Autodesk Inventor part; units mm, degrees
ref_plane "YZ Plane" through (0, 0, 0) normal (1, 0, 0) x (0, 1, 0)
ref_plane "XZ Plane" through (0, 0, 0) normal (0, 1, 0) x (-1, 0, 0)
ref_plane "XY Plane" through (0, 0, 0) normal (0, 0, 1) x (1, 0, 0)
sketch "Sketch1" plane through (0, 0, 0) normal (1, 0, 0) x (0, 1, 0)
  arc A0 (8.8122, -5.4272) -> (7.5394, -4.9) centre (7.5394, -6.7) ccw
  line L0 (8.8122, -5.4272) -> (10.3168, -6.9318)
  arc A1 (9.9986, -7.7) -> (10.3168, -6.9318) centre (9.9986, -7.25) ccw
  line L1 (9.9986, -7.7) -> (8.8, -7.7)
  arc A2 (8.8, -7.7) -> (8.5, -8) centre (8.8, -8) ccw
  line L2 (8.5, -8) -> (8.5, -8.1257)
  arc A3 (8.5, -8.1257) -> (8.5879, -8.3379) centre (8.8, -8.1257) ccw
  line L3 (8.5879, -8.3379) -> (9.25, -9)
  line L4 (9.25, -9) -> (18, -9)
  line L5 (4.75, -9) -> (5.4121, -8.3379)
  arc A4 (5.4121, -8.3379) -> (5.5, -8.1257) centre (5.2, -8.1257) ccw
  line L6 (5.5, -8.1257) -> (5.5, -8)
  arc A5 (5.5, -8) -> (5.2, -7.7) centre (5.2, -8) ccw
  line L7 (5.2, -7.7) -> (4.0014, -7.7)
  arc A6 (3.6832, -6.9318) -> (4.0014, -7.7) centre (4.0014, -7.25) ccw
  line L8 (3.6832, -6.9318) -> (5.1878, -5.4272)
  arc A7 (6.4606, -4.9) -> (5.1878, -5.4272) centre (6.4606, -6.7) ccw
  line L9 (6.4606, -4.9) -> (7.5394, -4.9)
  line L10 (-4.75, -9) -> (4.75, -9)
  line L11 (-5.4121, -8.3379) -> (-4.75, -9)
  arc A8 (-5.5, -8.1257) -> (-5.4121, -8.3379) centre (-5.2, -8.1257) ccw
  arc A9 (-5.2, -7.7) -> (-5.5, -8) centre (-5.2, -8) ccw
  line L12 (-4.0014, -7.7) -> (-5.2, -7.7)
  arc A10 (-4.0014, -7.7) -> (-3.6832, -6.9318) centre (-4.0014, -7.25) ccw
  line L13 (-5.1878, -5.4272) -> (-3.6832, -6.9318)
  arc A11 (-5.1878, -5.4272) -> (-6.4606, -4.9) centre (-6.4606, -6.7) ccw
  line L14 (-7.5394, -4.9) -> (-6.4606, -4.9)
  arc A12 (-7.5394, -4.9) -> (-8.8122, -5.4272) centre (-7.5394, -6.7) ccw
  line L15 (-10.3168, -6.9318) -> (-8.8122, -5.4272)
  line L16 (-18, -9) -> (-9.25, -9)
  line L17 (-9.25, -9) -> (-8.5879, -8.3379)
  line L18 (-5.5, -8) -> (-5.5, -8.1257)
  line L19 (-8.5, -8.1257) -> (-8.5, -8)
  arc A13 (-8.5879, -8.3379) -> (-8.5, -8.1257) centre (-8.8, -8.1257) ccw
  arc A14 (-8.5, -8) -> (-8.8, -7.7) centre (-8.8, -8) ccw
  line L20 (-8.8, -7.7) -> (-9.9986, -7.7)
  arc A15 (-10.3168, -6.9318) -> (-9.9986, -7.7) centre (-9.9986, -7.25) ccw
  line L21 (18, -9) -> (21, -9)
  line L22 (21, -9) -> (21, -14)
  line L23 (-18, -9) -> (-21, -9)
  line L24 (-21, -9) -> (-21, -14)
  line L25 (-21, -14) -> (21, -14)
  line L26 (21, -14) -> (31, -14)
  line L27 (31, -14) -> (31, -9)
  line L28 (31, -9) -> (21, -9)
  line L29 (-21, -14) -> (-31, -14)
  line L30 (-31, -14) -> (-31, -9)
  line L31 (-31, -9) -> (-21, -9)
  line L32 (-21, -14) -> (-21, -9)
  line L33 (21, -14) -> (21, -9)
  point P0 (0, 0)
  dimension "d0" = 5
  dimension "d7" = 10
  dimension "d9" = 10
extrude "Extrusion1" add sketch "Sketch1" along normal blind 456.6 contours L0 A1 L1 A2 L2 A3 L3 L4 L21 L22 L25 L24 L23 L16 L17 A13 L19 A14 L20 A15 L15 A12 L14 A11 L13 A10 L12 A9 L18 A8 L11 L10 L5 A4 L6 A5 L7 A6 L8 A7 L9 A0
sketch "Sketch2" plane through (0, 0, 0) normal (-1, 0, 0) x (0, 0, 1)
  circle A0 centre (-4.25, 15.7) radius 2.5
  circle A1 centre (28.25, 15.7) radius 2.5
  circle A2 centre (12, -0.55) radius 11
  circle A3 centre (28.25, -16.8) radius 2.5
  circle A4 centre (-4.25, -16.8) radius 2.5
  line L0 (-14, -21) -> (-14, 21)
  line L1 (-14, -21) -> (-9, -21)
  line L2 (-9, 21) -> (-14, 21)
  line L3 (-14, 21) -> (-14, -21)
  line L4 (33.45, 21) -> (33.45, -21)
  line L5 (33.45, -21) -> (-9.45, -21)
  line L6 (-9.45, 21) -> (33.45, 21)
  line L7 (-9, -9.25) -> (-9, -21)
  line L8 (33.45, -21) -> (-9, -21)
  line L9 (-13.9998, -20.9997) -> (-13.9998, -30.9997)
  line L10 (-9, -31) -> (33.45, -31)
  line L11 (33.45, -31) -> (33.45, -21)
  line L12 (33.45, 21) -> (-9, 21)
  line L13 (-14, 21) -> (-9, 21)
  line L14 (-13.9998, 21.0003) -> (-13.9998, 31.0003)
  line L15 (-9, 31) -> (33.45, 31)
  line L16 (33.45, 31) -> (33.45, 21)
  line L17 (-13.9998, -30.9997) -> (33.45, -30.9997)
  line L18 (33.45, -30.9997) -> (33.45, -21)
  line L19 (33.45, -21) -> (-13.9998, -21)
  line L20 (-13.9998, -21) -> (-13.9998, -30.9997)
  line L21 (33.45, 21) -> (-13.9998, 21)
  line L22 (-13.9998, 21) -> (-13.9998, 31.0003)
  line L23 (-13.9998, 31.0003) -> (33.45, 31.0003)
  line L24 (33.45, 31.0003) -> (33.45, 21)
  point P0 (12, -11.55)
  point P1 (-14, 21)
  point P2 (-13.9998, -21)
  dimension "d12" = 11.18
  dimension "d13" = 11.1805
extrude "Extrusion2" add sketch "Sketch2" along normal blind 5 contours L0 L2 L6 L4 L5 L1
extrude "Extrusion3" add sketch "Sketch1" along normal up to surface (456.6 mm away) contours L28 L27 L26 L22 | L29 L30 L31 L24
extrude "Extrusion4" add sketch "Sketch2" along normal up to surface (5 mm away) contours L1 L5 L11 L10 L17 L9 | L14 L23 L15 L16 L6 L2
sketch "Sketch3" plane through (-5, -21, -14) normal (0, 0, -1) x (-1, 0, 0)
  line L0 (-461.6, -10) -> (-461.6, 0)
  line L1 (-461.6, -10) -> (-451.6, -10)
  line L2 (-451.6, -10) -> (-451.6, 0)
  line L3 (-451.6, 0) -> (-461.6, 0)
  line L4 (-461.6, 0) -> (-461.6, -10)
  line L5 (-5, -10) -> (-461.6, -10)
  line L6 (-461.6, -10) -> (-451.6, 0)
  line L7 (-5, 0) -> (-461.6, 0)
  line L8 (-461.6, 0) -> (-451.6, -10)
  circle A0 centre (-456.6, -5) radius 2.5
  line L9 (-5, 52) -> (-461.6, 52)
  line L10 (-461.6, 52) -> (-451.6, 52)
  line L11 (-451.6, 52) -> (-451.6, 42)
  line L12 (-451.6, 42) -> (-461.6, 42)
  line L13 (-461.6, 42) -> (-461.6, 52)
  line L14 (-461.6, 42) -> (-451.6, 52)
  line L15 (-461.6, 52) -> (-451.6, 42)
  circle A1 centre (-456.6, 47) radius 2.5
  line L16 (0, -9.9997) -> (0, 0)
  line L17 (0, -9.9997) -> (-20, -9.9997)
  line L18 (-20, -9.9997) -> (-20, 0.0003)
  line L19 (-20, 0.0003) -> (0, 0.0003)
  line L20 (0, 0.0003) -> (0, -9.9997)
  line L21 (-5, 0) -> (0, 0)
  line L22 (-20, -9.9997) -> (0, 0)
  line L23 (0, 0) -> (-20, 0.0003)
  line L24 (-20, 0.0003) -> (0, -9.9997)
  circle A2 centre (-10, -4.9997) radius 2.5
  line L25 (0, 52.0003) -> (0, -9.9997)
  line L26 (0, 52.0003) -> (-20, 52.0003)
  line L27 (-20, 52.0003) -> (-20, 42.0003)
  line L28 (-20, 42.0003) -> (0, 42.0003)
  line L29 (0, 42.0003) -> (0, 52.0003)
  line L30 (-20, 42.0003) -> (0, 52.0003)
  line L31 (-20, 52.0003) -> (0, 42.0003)
  circle A3 centre (-10, 47.0003) radius 2.5
  point P0 (-5, 21)
  dimension "d22" = 10
  dimension "d23" = 10
  dimension "d24" = 5
  dimension "d25" = 10
  dimension "d26" = 10
  dimension "d27" = 5
  dimension "d28" = 20
  dimension "d29" = 10
  dimension "d30" = 5
  dimension "d31" = 20
  dimension "d32" = 10
  dimension "d33" = 5
extrude "Extrusion5" cut sketch "Sketch3" against normal through all contours A0 L8 L6 | L6 L8 A0 | A0 L6 L8 | L8 L6 A0 | A2 L24 L22 | L22 L24 A2 | A2 L22 L24 | L22 A2 L24 | A3 L30 L31 | L31 L30 A3 | L30 L31 A3 | A3 L31 L30 | A1 L15 L14 | L14 L15 A1 | L15 L14 A1 | A1 L14 L15
properties part number "SoporteElectromecánico" material "Steel, Mild, Welded"
The listing builds one solid part. Answer for the finished solid, in the listing's coordinates (mm). Give positions to 0.01 mm unless a question says otherwise; leave off trailing zeros. Order: outer loops, then holes, each group sorted by start corner. A loop starts at its lowest first (then second) coordinate and runs counter-clockwise, first axis right, second up. Notation, with made-up numbers: (-5, -22.5) - (41, -22.5) arc R7 ccw to (41, -15.5) - close; hole circle Ø3 at (24, 87). An arc over 180 degrees is marked (long way). Answer as CSV lines item,"result".
Q1. Each of these flat-tipped pins is pushed along its axis until it touches: pin 1 Ø3 at (x, y) = (92.5, 23) entering from +Z; pin 2 Ø5 at (x, z) = (388.5, -1.5) entering from +Y; pin 3 Ø8 at (y, z) = (15.7, -4.25) entering from +X. Where does it stop, or does it pass through?
Answer key:
pin 1,"stops at z = -9"
pin 2,"passes through"
pin 3,"stops at x = 0"
Q2. Straight lines are drawn through the part: L1, parallel to X at y = 26, z = -12; L2, parallel to Y at x = -3, z = 28; L3, parallel to X at y = 3.5, z = -1.5. For each, find the intervals that lie inside material, in ascending order.
Answer key:
L1,"x = -5 to 2.5, 7.5 to 449.1, 454.1 to 456.6"
L2,"y = -31 to -19.29, -14.31 to 13.21, 18.19 to 31"
L3,"x = -5 to 0"
Q3. A cutting plane is placed at A-A, the plane z = 7.5. Determine the outline of the cut face in (x, y).
Answer key:
outline,"(-5, -31) - (0, -31) - (0, -10.59) - (-5, -10.59) - close; (-5, 9.49) - (0, 9.49) - (0, 31) - (-5, 31) - close"
Q4. Determine the mould class of faces 1 (the face through (225, 0, -9)), 2 (the face through (-2.465, 3.663, 22.161)), 3 (the face through (456.6, 0, -10)) for opening direction Y: pulls with the +Y half, pulls with the -Y half, needs draft (parallel to the pull), parting line crosses it, or undercut.
Answer key:
face 1,"undercut"
face 2,"undercut"
face 3,"needs draft"
